Could you check a few things on this model? Use its own coordinates, in mm. Face numbers are marked on the shaded views. Give positions to 0.01 mm unless a question says otherwise; leave off trailing zeros. Write each loop counter-clockwise with the first axis right and the second up, starting at its lowest first coordinate (ties: lowest second). Pieces come first, ordered by that corner, then holes. Notation, with made-up numbers: (57, -26.5) - (88, -26.5) arc R22 cw to (88, -10.5) - close; hole circle Ø8 at (13, 55). An arc over 180 degrees is marked (long way). Write item = value, one per line.
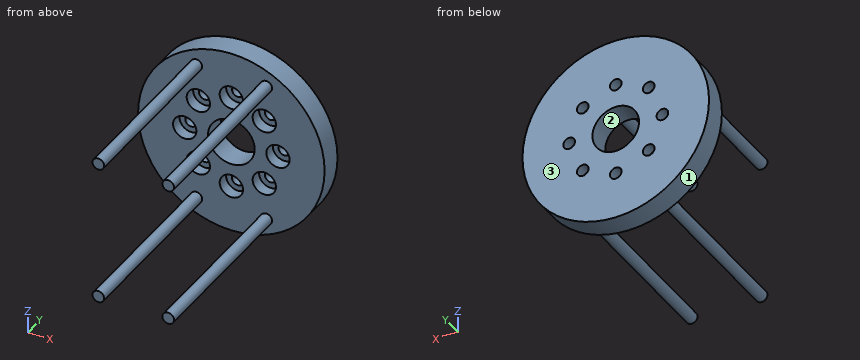
from build123d import *

# Parameters (mm, degrees)
F0_R           = 50.8
F0_R_2         = 12.7
F1_DEPTH       = 12.7
F2_R           = 6.35
F3_DEPTH       = 6.35
F4_D           = 6.35
F4_CBORE_D     = 12.7
F4_CBORE_DEPTH = 6.35
F5_R           = 3.175
F6_DEPTH       = 96.52
F7_R           = 3.175
F8_DEPTH       = 25.4


with BuildPart() as f1:
    # F0 (on Front) → F1 (new body)
    with BuildSketch(Plane.XZ):
        Circle(F0_R)
        Circle(F0_R_2, mode=Mode.SUBTRACT)
    extrude(amount=F1_DEPTH)

    # F2 (on face) → F3 (cut)
    with BuildSketch(Plane.XZ.offset(12.7)):
        with Locations((-17.960512, 17.960512)):
            Circle(F2_R)
        with Locations((17.960512, 17.960512)):
            Circle(F2_R)
        with Locations((17.960512, -17.960512)):
            Circle(F2_R)
        with Locations((-17.960512, -17.960512)):
            Circle(F2_R)
    extrude(amount=-F3_DEPTH, mode=Mode.SUBTRACT)

    # F4 (through all)
    with Locations(Plane.XZ.offset(12.7)):
        with Locations((0, 25.4), (-25.4, 0), (0, -25.4), (25.4, 0)):
            CounterBoreHole(F4_D / 2, F4_CBORE_D / 2, F4_CBORE_DEPTH)

    # F5 (on face) → F6 (join)
    with BuildSketch(Plane.XZ.offset(12.7)):
        with Locations((-19.05, 38.1)):
            Circle(F5_R)
        with Locations((19.05, 38.1)):
            Circle(F5_R)
        with Locations((19.05, -38.1)):
            Circle(F5_R)
        with Locations((-19.05, -38.1)):
            Circle(F5_R)
    extrude(amount=F6_DEPTH)

    # F7 (on face) → F8 (cut)
    with BuildSketch(Plane.XZ.offset(6.35)):
        with Locations((-17.960512, 17.960512)):
            Circle(F7_R)
        with Locations((-17.960512, -17.960512)):
            Circle(F7_R)
        with Locations((17.960512, 17.960512)):
            Circle(F7_R)
        with Locations((17.960512, -17.960512)):
            Circle(F7_R)
    extrude(amount=-F8_DEPTH, mode=Mode.SUBTRACT)


solid = f1.part
1. If we section it at A-A, the plane x = 0: Please give me the cut outline in (y, z) (3 decimals).
Filled sheet:
outline = (-12.7, -50.8) - (0, -50.8) - (0, -28.575) - (-6.35, -28.575) - (-6.35, -31.75) - (-12.7, -31.75) - close; (-12.7, -19.05) - (-6.35, -19.05) - (-6.35, -22.225) - (0, -22.225) - (0, -12.7) - (-12.7, -12.7) - close; (-12.7, 12.7) - (0, 12.7) - (0, 22.225) - (-6.35, 22.225) - (-6.35, 19.05) - (-12.7, 19.05) - close; (-12.7, 31.75) - (-6.35, 31.75) - (-6.35, 28.575) - (0, 28.575) - (0, 50.8) - (-12.7, 50.8) - close
2. For pin 1 (11.5 mm diameter, centred on x = 17.96, z = 17.96, fed in from -Y); pin 2 (2 mm diameter, centred on x = -2, z = 40.5, fed in from -Y); pin 3 (10 mm diameter, centred on x = -31, y = -24, fed in from -Z); pin 4 (3 mm diameter, centred on y = -73, z = 36.5, fed in from +X), each with a flat end and sliding along its axis, tell me the tip position at first contact or that it passes through.
Filled sheet:
pin_1 = -6.35
pin_2 = -12.7
pin_3 = through
pin_4 = 22.22
3. If we section it at D-D, the plane x = 35.5: Please give me the cut outline in (y, z).
Filled sheet:
outline = (-12.7, -36.34) - (0, -36.34) - (0, 36.34) - (-12.7, 36.34) - close
4. If we section it at B-B, the plane y = -23: Please give me the cut outline in (x, z) (3 decimals).
Filled sheet:
outline = circle Ø6.35 at (-19.05, -38.1); circle Ø6.35 at (-19.05, 38.1); circle Ø6.35 at (19.05, -38.1); circle Ø6.35 at (19.05, 38.1)
5. Thinking about a two-plate mould opening in X: for the marked faces 1, 2 and 3, which applies, pulls with the +X half, pulls with the -X half, needs draft (parallel to the pull), parting line crosses it, or undercut?
Filled sheet:
face_1 = parting line crosses it
face_2 = undercut
face_3 = needs draft
6. I need wall thicknesses on line 1 (Z direction, x = 0, y = -10); line 2 (Z direction, x = 0, y = -1.5) (3 decimals); line 3 (Z direction, x = 18.5, y = -10.5). Which ranges of each line are inside material? Lowest first, please.
Filled sheet:
line_1 = -50.8 to -31.75, -19.05 to -12.7, 12.7 to 19.05, 31.75 to 50.8
line_2 = -50.8 to -28.575, -22.225 to -12.7, 12.7 to 22.225, 28.575 to 50.8
line_3 = -47.31 to -24.29, -11.63 to 11.63, 24.29 to 47.31
7. If we section it at C-C, the plane z = -38.1: Please give me the cut outline in (x, y) (3 decimals), and give its area (3 significant figures).
Filled sheet:
outline = (-33.601, -12.7) - (-22.225, -12.7) - (-22.225, -109.22) - (-15.875, -109.22) - (-15.875, -12.7) - (15.875, -12.7) - (15.875, -109.22) - (22.225, -109.22) - (22.225, -12.7) - (33.601, -12.7) - (33.601, 0) - (-33.601, 0) - close
area = 2,080 mm2
